Autodesk Fusion 360 part; units mm, degrees
sketch "Sketch9" plane through (0, 0, 0) normal (0, 0, 1) x (1, 0, 0)
  line L0 (0, 50) -> (50, 50)
  line L1 (50, 50) -> (50, 0)
  line L2 (50, 0) -> (0, 0)
  line L3 (0, 0) -> (0, 50)
  line L4 (-25, 50) -> (0, 50)
  line L5 (0, 50) -> (0, 0)
  line L6 (0, 0) -> (-25, 0)
  line L7 (-25, 0) -> (-25, 50)
  line L8 (50, 50) -> (75, 50)
  line L9 (75, 50) -> (75, 0)
  line L10 (75, 0) -> (50, 0)
  line L11 (50, 0) -> (50, 50)
  dimension "d34" = 50
  dimension "d35" = 50
  dimension "d36" = 25
  dimension "d37" = 50
extrude "Extrude5" add sketch "Sketch9" along normal blind 30 contours L0 L1 L2 L3 L5 L11
extrude "Extrude6" add sketch "Sketch9" along normal blind 5 contours L1 L8 L9 L10 L11
extrude "Extrude7" add sketch "Sketch9" along normal blind 5 contours L3 L4 L5 L6 L7
sketch "Sketch12" plane through (0, 0, 0) normal (0, 1, 0) x (1, 0, 0)
  line L0 (5, -25) -> (45, -25)
  line L1 (45, -25) -> (45, 0)
  line L2 (45, 0) -> (5, 0)
  line L3 (5, 0) -> (5, -25)
  line L4 (50, 0) -> (0, 0)
  line L5 (75, 0) -> (-25, 0)
  line L6 (-25, 0) -> (75, 0)
  line L7 (0, -30) -> (50, -30)
  line L8 (0, -5) -> (0, -30)
  line L9 (50, -5) -> (50, -30)
  dimension "d44" = 5
  dimension "d45" = 5
  dimension "d46" = 5
extrude "Extrude8" cut sketch "Sketch12" along normal through all
sketch "Sketch13" plane through (0, 0, 30) normal (0, 0, 1) x (-1, 0, 0)
  line L0 (0, -50) -> (0, 0)
  line L1 (0, 0) -> (-50, 0)
  line L2 (-50, 0) -> (-50, -50)
  line L3 (-50, -50) -> (0, -50)
  circle A0 centre (-25, -12.5) radius 2.25
  circle A1 centre (-25, -37.5) radius 2.25
  dimension "d48" = 4.5
  dimension "d49" = 4.5
  dimension "d50" = 25
  dimension "d51" = 25
  dimension "d52" = 12.5
extrude "Extrude9" cut sketch "Sketch13" against normal through all contours A0
extrude "Extrude10" cut sketch "Sketch13" against normal through all contours A1
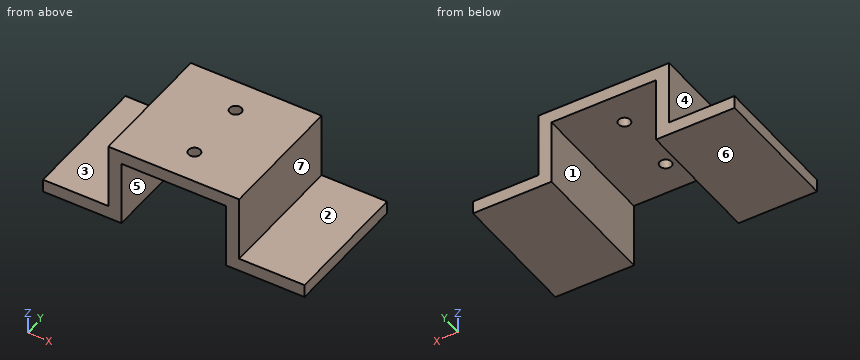
For this review, take the finished solid that the model builds, in its own axes (mm). Face numbers are marked on the shaded views. A direction names the side the tool comes from. Round coordinates to 2 decimals unless told otherwise and drop trailing zeros. Write each loop counter-clockwise with the first axis right and the second up, starting at its lowest first coordinate (ties: lowest second). Pieces come first, ordered by that corner, then holes. Notation, with made-up numbers: (84, 24.25) -> (97, 24.25) arc R21 ccw to (97, 60.25) -> close; hole circle Ø5 at (-22, 57.25). An arc over 180 degrees is marked (long way). Use CSV: the item, a comma, the result in double quotes.
(1) Consider section A-A, the plane x = 25. Give the boundary of the cut face in (y, z).
Computed values:
outline,"(0, 25) -> (10.25, 25) -> (10.25, 30) -> (0, 30) -> close; (14.75, 25) -> (35.25, 25) -> (35.25, 30) -> (14.75, 30) -> close; (39.75, 25) -> (50, 25) -> (50, 30) -> (39.75, 30) -> close"
(2) Consider section D-D, the plane y = 43. Give the boundary of the cut face in (x, z).
Computed values:
outline,"(-25, 0) -> (5, 0) -> (5, 25) -> (45, 25) -> (45, 0) -> (75, 0) -> (75, 5) -> (50, 5) -> (50, 30) -> (0, 30) -> (0, 5) -> (-25, 5) -> close"
(3) Consider section C-C, the plane z = 11.75. Give the boundary of the cut face in (x, y).
Computed values:
outline,"(0, 0) -> (5, 0) -> (5, 50) -> (0, 50) -> close; (45, 0) -> (50, 0) -> (50, 50) -> (45, 50) -> close"
(4) For the marked faces 1, 2 and 3, list the 3-axis set-ups (+Z, -Z, +X, -X, +Y, -Y) from which the entire face can be reached by the end or side of a thin tool; tool diameter is ignored.
Computed values:
face 1,"-Z, +Y, -Y"
face 2,"+Z, +X, +Y, -Y"
face 3,"+Z, -X, +Y, -Y"
(5) Consider section B-B, the plane y = 37.5. Give the boundary of the cut face in (x, z).
Computed values:
outline,"(-25, 0) -> (5, 0) -> (5, 25) -> (22.75, 25) -> (22.75, 30) -> (0, 30) -> (0, 5) -> (-25, 5) -> close; (27.25, 25) -> (45, 25) -> (45, 0) -> (75, 0) -> (75, 5) -> (50, 5) -> (50, 30) -> (27.25, 30) -> close"
(6) Draft analysis for pull direction X (two halves, no side actions). For the marked faces 4, 5, 6 and 7, state which applies: +X half, -X half, draft (parallel to the pull), parting line (faces both ways), or undercut.
Computed values:
face 4,"-X half"
face 5,"undercut"
face 6,"draft"
face 7,"+X half"
(7) To check wall thickness, follow L1, parallel to Y at x = 25, z = 26.15; L2, parallel to X at y = 15.5, z = 22; L3, parallel to X at y = 37.5, z = 26.35. State the ranges of each line that lie inside material, in increasing order. Write a range as [from, to].
Computed values:
L1,"[0, 10.25], [14.75, 35.25], [39.75, 50]"
L2,"[0, 5], [45, 50]"
L3,"[0, 22.75], [27.25, 50]"
(8) Clearance check with flat-ended pins moving along their axes: P1, Ø1, axis at y = 14.5, z = 14.5, coming from the +X side; P2, Ø3.5, axis at x = 25, y = 37.5, coming from the +Z side (3 decimals); P3, Ø3, axis at x = 18, y = 11.5, coming from the -Z side; P4, Ø7.5, axis at x = 66, y = 19, coming from the +Z side. State where each tip first meets the part, or that it passes through.
Computed values:
P1,"x = 50"
P2,"through"
P3,"z = 25"
P4,"z = 5"
